Geometry: final body of the model. Coordinates: model frame, mm. A direction names the side the tool comes from. Give positions to 0.01 mm unless a question says otherwise; leave off trailing zeros. Write each loop counter-clockwise with the first axis right and the second up, starting at its lowest first coordinate (ties: lowest second). Pieces come first, ordered by that corner, then holes. Notation, with made-up numbers: (-23.75, -37.5) -> (-12.75, -37.5) arc R14 cw to (-12.75, -17.5) -> close; hole circle Ø10 at (75, 89). An arc over 180 degrees is marked (long way). Answer in a Markdown table with one row per item. Add a question column.
Item 1: Section query B-B on y = -45.5. Output: boundary loops of the cut face in (x, z), plus the area to 3 significant figures.
Item 2: First-contact query: P1, Ø1.2, axis at y = -101, z = -1.5, coming from the +X side; P2, Ø4, axis at y = -8.5, z = 27, coming from the +X side; P3, Ø1, axis at y = -40, z = -10.5, coming from the +X side. Flat tips, straight axial feed; report the tip coordinate or a pass-through.
Item 3: Section query C-C on x = 89. Output: boundary loops of the cut face in (y, z).
Item 4: Section query D-D on z = -17. Output: boundary loops of the cut face in (x, y).
Item 5: Access query for faces 4 (the flat face through (100, 20, 4)), 5 (the flat face through (38, -18, 80)). Directions: +Z, -Z, +X, -X, +Y, -Y. A direction counts if a zero-diameter tool reaches every point of the face in a straight line with its end or side. Return the directions, or none.
Item 6: Material intervals for probe 1 along Z at (x, y) = (37, 32); probe 2 along Y at (x, z) = (28.5, -7.5); probe 3 along Y at (x, z) = (88.5, -1), sorted ascending. Write a range as from..to.
Item 7: Section query A-A on z = 9. Output: boundary loops of the cut face in (x, y).
Item 8: Draft query along Z for faces 1 (the flat face through (38, -18, 81)), 2 (the flat face through (38, -18, -75)), 3 (the flat face through (99, 20, 4)). Return one class per face: +Z half, -Z half, draft (parallel to the pull), parting line (faces both ways), or undercut.
```python
from build123d import *

# Parameters (mm, degrees)
ESQUISSE1_W              = 156
ESQUISSE1_H              = 156
BOSS_EXTRU_3_DEPTH       = 100
ESQUISSE5_W              = 75
ESQUISSE5_H              = 26
ENL_V_MAT_EXTRU_4_DEPTH  = 100
ENL_V_MAT_EXTRU_11_DEPTH = 217.60592354
COQUE6_T                 = -1
ENL_V_MAT_EXTRU_12_REACH = 178.199


with BuildPart() as part:
    # Esquisse1 → Boss.-Extru.3 (new body)
    with BuildSketch(Plane(origin=(0, 0, 0), x_dir=(0, 0, -1), z_dir=(1, 0, 0))):
        with Locations((-3, -34.170076726)):
            Rectangle(ESQUISSE1_W, ESQUISSE1_H)
    extrude(amount=BOSS_EXTRU_3_DEPTH)

    # Esquisse5 → Enlèv. mat.-Extru.4 (cut)
    with BuildSketch(Plane.XZ.offset(112.170076726)):
        with Locations((47.5, 3)):
            Rectangle(ESQUISSE5_W, ESQUISSE5_H)
    extrude(amount=-ENL_V_MAT_EXTRU_4_DEPTH, mode=Mode.SUBTRACT)

    # Esquisse8 → Enlèv. mat.-Extru.11 (cut, through all)
    with BuildSketch(Plane.XY.offset(81)):
        Polygon((100, -4.709521913), (0, -112.170076726), (100, -112.170076726), align=None)
    extrude(amount=-ENL_V_MAT_EXTRU_11_DEPTH, mode=Mode.SUBTRACT)

    # Coque6
    coque6_openings = [part.faces().sort_by_distance(p)[0] for p in [
        (0, -34.170076726, 3),
    ]]
    offset(amount=COQUE6_T, openings=coque6_openings, kind=Kind.INTERSECTION)

    # Esquisse10 → Enlèv. mat.-Extru.12 (cut, up to next)
    with BuildSketch(Plane(origin=(0, 0, -11), x_dir=(-1, 0, 0), z_dir=(0, 0, -1)), mode=Mode.PRIVATE) as enl_v_mat_extru_12_sk1:
        Polygon((-9, -101.030710895), (-86, -18.286083689), (-86, -11.170076726), (-9, -11.170076726), align=None)
    enl_v_mat_extru_12_tool1 = extrude(enl_v_mat_extru_12_sk1.sketch, amount=-ENL_V_MAT_EXTRU_12_REACH, mode=Mode.PRIVATE) & part.part
    add(enl_v_mat_extru_12_tool1.solids().sort_by_distance((36.55005, -41.297676, -11))[0], mode=Mode.SUBTRACT)


solid = part.part
```
Findings below:
| question | item | result |
|---|---|---|
| 1 | outline | (0, -75) -> (62.04, -75) -> (62.04, -10) -> (60.68, -10) -> (60.68, -74) -> (0, -74) -> close; (0, 80) -> (60.68, 80) -> (60.68, 16) -> (62.04, 16) -> (62.04, 81) -> (0, 81) -> close |
| 1 | area | 299 mm^2 |
| 2 | P1 | stops at x = 10 |
| 2 | P2 | stops at x = 98.33 |
| 2 | P3 | stops at x = 67.62 |
| 3 | outline | (-16.53, -75) -> (43.83, -75) -> (43.83, 81) -> (-16.53, 81) -> close; hole (-15.06, -74) -> (42.83, -74) -> (42.83, 80) -> (-15.06, 80) -> close |
| 4 | outline | (0, -112.17) -> (100, -4.71) -> (100, 43.83) -> (0, 43.83) -> (0, 42.83) -> (99, 42.83) -> (99, -4.32) -> (0, -110.7) -> close |
| 5 | face 4 | +Z, -Z, +X, +Y, -Y |
| 5 | face 5 | -X |
| 6 | probe 1 | z = -75..-74, 80..81 |
| 6 | probe 2 | y = 42.83..43.83 |
| 6 | probe 3 | y = -17.07..-15.6, 42.83..43.83 |
| 7 | outline | (0, -112.17) -> (10, -101.42) -> (10, -99.96) -> (0, -110.7) -> close; (0, 42.83) -> (99, 42.83) -> (99, -4.32) -> (85, -19.36) -> (85, -20.83) -> (100, -4.71) -> (100, 43.83) -> (0, 43.83) -> close |
| 8 | face 1 | +Z half |
| 8 | face 2 | -Z half |
| 8 | face 3 | undercut |
